```python
from build123d import *

# Parameters (mm, degrees)
F1_DEPTH = 1016


with BuildPart() as f1:
    # F0 (on Front) → F1 (new body)
    with BuildSketch(Plane.XZ):
        with BuildLine():
            Line((-1393.375381, -25.4), (-1393.375381, -254))
            Line((-1393.375381, -254), (-453.575381, -254))
            Line((-453.575381, -254), (-453.575381, 101.6))
            Line((-453.575381, 101.6), (3.624619, 101.6))
            Line((3.624619, 101.6), (3.624619, -254))
            Line((3.624619, -254), (943.424619, -254))
            Line((943.424619, -254), (943.424619, -25.4))
            Line((943.424619, -25.4), (257.624619, -25.4))
            ThreePointArc((257.624619, -25.4), (239.664107, -17.960512), (232.224619, 0))
            Line((232.224619, 0), (232.224619, 304.8))
            ThreePointArc((232.224619, 304.8), (224.785132, 322.760512), (206.824619, 330.2))
            Line((206.824619, 330.2), (-656.775381, 330.2))
            ThreePointArc((-656.775381, 330.2), (-674.735893, 322.760512), (-682.175381, 304.8))
            Line((-682.175381, 304.8), (-682.175381, 0))
            ThreePointArc((-682.175381, 0), (-689.614868, -17.960512), (-707.575381, -25.4))
            Line((-707.575381, -25.4), (-1393.375381, -25.4))
        make_face()
    extrude(amount=F1_DEPTH)


solid = f1.part
```
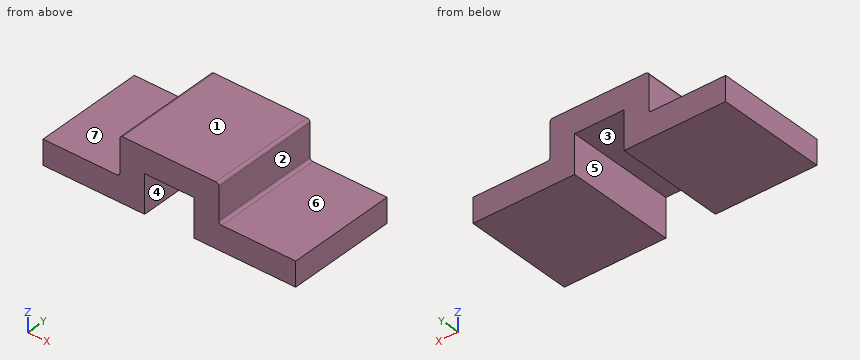
Design review of the part built by this model. Coordinates are the model's own, in mm. Face numbers are marked on the shaded views. A direction names the side the tool comes from. Coordinates: 2 decimals unless noted, no trailing zeros. Write each loop counter-clockwise with the first axis right and the second up, starting at its lowest first coordinate (ties: lowest second). Pieces come first, ordered by that corner, then holes. Notation, with made-up numbers: M -29,70 L 20,70 A12 ccw 20,85 Z; hole C -2.5,84.25 d2. An arc over 180 degrees is marked long. Answer as a JSON object with one key per item and string values.
Item 1: Add section C-C, the plane x = -411. Give the boundary of the cut face in (y, z), and give its area (3 significant figures).
Outcome:
{"outline": "M -1016,101.6 L 0,101.6 L 0,330.2 L -1016,330.2 Z", "area": "232,000 mm²"}
Item 2: Add section A-A, the plane z = -185. Give the boundary of the cut face in (x, y).
Outcome:
{"outline": "M -1393.38,-1016 L -453.58,-1016 L -453.58,0 L -1393.38,0 Z; M 3.62,-1016 L 943.42,-1016 L 943.42,0 L 3.62,0 Z"}
Item 3: Machinability: for the marked faces 5, 6 and 7, which of the approach directions +Z, -Z, +X, -X, +Y, -Y give a long, thin tool a straight path to every point of the face, cutting with its end or side? Answer none if there is none.
Outcome:
{"face 5": "-Z, +Y, -Y", "face 6": "+Z, +X, +Y, -Y", "face 7": "+Z, -X, +Y, -Y"}
Item 4: Insertion check: pin 1 Ø2 at (x, y) = (-100.5, -521.5) entering from -Z; pin 2 Ø10 at (x, y) = (503.5, -148) entering from +Z. Each pin has a flat end and moves straight along its axis. Give the tip position at first contact, or say it passes through.
Outcome:
{"pin 1": "z = 101.6", "pin 2": "z = -25.4"}
Item 5: Wall thickness on probe 1 along X at (y, z) = (-658, 59); probe 2 along X at (y, z) = (-405.5, -46); probe 3 along Z at (x, y) = (-180, -880): over which ranges is each line inside the solid? List them lowest first.
Outcome:
{"probe 1": "-682.18 to -453.58, 3.62 to 232.22", "probe 2": "-1393.38 to -453.58, 3.62 to 943.42", "probe 3": "101.6 to 330.2"}
Item 6: Draft analysis for pull direction X (two halves, no side actions). For the marked faces 1, 2, 3 and 4, state which applies: pulls with the +X half, pulls with the -X half, needs draft (parallel to the pull), parting line crosses it, or undercut.
Outcome:
{"face 1": "needs draft", "face 2": "pulls with the +X half", "face 3": "undercut", "face 4": "undercut"}
Item 7: Add section B-B, the plane y = -495.5. Give the boundary of the cut face in (x, z).
Outcome:
{"outline": "M -1393.38,-254 L -453.58,-254 L -453.58,101.6 L 3.62,101.6 L 3.62,-254 L 943.42,-254 L 943.42,-25.4 L 257.62,-25.4 A25.4 cw 232.22,0 L 232.22,304.8 A25.4 ccw 206.82,330.2 L -656.78,330.2 A25.4 ccw -682.18,304.8 L -682.18,0 A25.4 cw -707.58,-25.4 L -1393.38,-25.4 Z"}
